from build123d import *

# Parameters (mm, degrees)
BOSS_EXTRUDE1_DEPTH      = 15
BOSS_EXTRUDE1_DEPTH_BACK = 15
SKETCH1_W                = 48
SKETCH1_H                = 65
SKETCH2_R                = 1.25
CUT_EXTRUDE1_DEPTH       = 10
SKETCH4_R                = 9.5
SKETCH4_R_2              = 8
SKETCH4_R_3              = 3
BOSS_EXTRUDE3_DEPTH      = 1.5
CHAMFER2_SIZE            = 1.5
SKETCH5_R                = 3
BOSS_EXTRUDE4_DEPTH      = 6
CHAMFER2_OF_MIRROR1_SIZE = 1.5
SKETCH6_R                = 1.25
SKETCH6_R_2              = 1.249999994
CUT_EXTRUDE2_DEPTH       = 10
FILLET1_R                = 2.5


with BuildPart() as part:
    # Sketch1 → Boss-Extrude1 (new, two sides: drawn at the far end of the back side and taken through both)
    with BuildSketch(Plane.XY.offset(-BOSS_EXTRUDE1_DEPTH_BACK)):
        Rectangle(SKETCH1_W, SKETCH1_H)
    extrude(amount=BOSS_EXTRUDE1_DEPTH + BOSS_EXTRUDE1_DEPTH_BACK)

    # Sketch2 → Cut-Extrude1 (cut)
    with BuildSketch(Plane.ZY.offset(24)):
        with Locations(Location((-12, 29.5, 0), (0, 0, 270))):
            Circle(SKETCH2_R)
        with Locations(Location((12, 29.5, 0), (0, 0, 270))):
            Circle(SKETCH2_R)
        with Locations(Location((12, 5.5, 0), (0, 0, 270))):
            Circle(SKETCH2_R)
        with Locations(Location((-12, 5.5, 0), (0, 0, 270))):
            Circle(SKETCH2_R)
        with Locations(Location((-12, -29.5, 0), (0, 0, 270))):
            Circle(SKETCH2_R)
        with Locations(Location((12, -29.5, 0), (0, 0, 270))):
            Circle(SKETCH2_R)
    extrude(amount=-CUT_EXTRUDE1_DEPTH, mode=Mode.SUBTRACT)

    # Sketch4 → Boss-Extrude3 (add)
    # profile 1 of 3: a face of its own
    with BuildSketch(Plane.ZY.offset(24)):
        with Locations(Location((0, 20.5, 0), (0, 0, 270))):
            Circle(SKETCH4_R)
        with Locations((0, 20.5)):
            Circle(SKETCH4_R_2, mode=Mode.SUBTRACT)
    # profile 2 of 3: a face of its own
    with BuildSketch(Plane.ZY.offset(24)):
        with Locations((0, 20.5)):
            Circle(SKETCH4_R_2)
        with Locations((0, 20.5)):
            Circle(SKETCH4_R_3, mode=Mode.SUBTRACT)
    # profile 3 of 3: a face of its own
    with BuildSketch(Plane.ZY.offset(24)):
        with Locations((0, 20.5)):
            Circle(SKETCH4_R_3)
    boss_extrude3 = extrude(amount=BOSS_EXTRUDE3_DEPTH)

    # Chamfer2
    chamfer2_edges = [part.edges().sort_by_distance(p)[0] for p in [
        (-25.5, 30, 0),
    ]]
    chamfer(chamfer2_edges, length=CHAMFER2_SIZE - 0.0001)  # a hair under: the kernel refuses the full size

    # Sketch5 → Boss-Extrude4 (add)
    with BuildSketch(Plane.ZY.offset(25.5)):
        with Locations(Location((0, 20.5, 0), (0, 0, 270))):
            Circle(SKETCH5_R)
    boss_extrude4 = extrude(amount=BOSS_EXTRUDE4_DEPTH)

    # Mirror1: Boss-Extrude3, Boss-Extrude4 across plane
    add(boss_extrude3.mirror(Plane(origin=(0, 0, 0), x_dir=(0, 0, 1), z_dir=(1, 0, 0))))
    add(boss_extrude4.mirror(Plane(origin=(0, 0, 0), x_dir=(0, 0, 1), z_dir=(1, 0, 0))))

    # Chamfer2 of Mirror1
    chamfer2_of_mirror1_edges = [part.edges().sort_by_distance(p)[0] for p in [
        (25.5, 30, 0),
    ]]
    chamfer(chamfer2_of_mirror1_edges, length=CHAMFER2_OF_MIRROR1_SIZE - 0.0001)  # a hair under: the kernel refuses the full size

    # Sketch6 → Cut-Extrude2 (cut)
    with BuildSketch(Plane(origin=(24, 0, 0), x_dir=(0, 0, -1), z_dir=(1, 0, 0))):
        with Locations(Location((11.99999998, -5, 0), (0, 0, 90))):
            Circle(SKETCH6_R)
        with Locations(Location((12.00000002, -17.5, 0), (0, 0, 90))):
            Circle(SKETCH6_R)
        with Locations(Location((0, -29.5, 0), (0, 0, 90))):
            Circle(SKETCH6_R_2)
        with Locations(Location((-12.00000002, -17.5, 0), (0, 0, 90))):
            Circle(SKETCH6_R)
        with Locations(Location((-12.00000002, 9.5, 0), (0, 0, 90))):
            Circle(SKETCH6_R)
    extrude(amount=-CUT_EXTRUDE2_DEPTH, mode=Mode.SUBTRACT)

    # Fillet1
    fillet1_edges = [part.edges().sort_by_distance(p)[0] for p in [
        (0, -32.5, 15),
        (0, 32.5, 15),
        (0, 32.5, -15),
        (0, -32.5, -15),
    ]]
    fillet(fillet1_edges, radius=FILLET1_R)


solid = part.part
Verification items for the finished model (mm, model axes). A direction names the side the tool comes from. Give positions to 0.01 mm unless a question says otherwise; leave off trailing zeros. Write each loop counter-clockwise with the first axis right and the second up, starting at its lowest first coordinate (ties: lowest second). Pieces come first, ordered by that corner, then holes. Notation, with made-up numbers: M -13.75,40.25 L 20.25,40.25 A34 ccw 20.25,70.25 Z; hole C 11,44.25 d3. An arc over 180 degrees is marked long. Write item = value, one per line.
(1) Material ranges on line 1 (Z direction, x = 21, y = -17.5); line 2 (X direction, y = 4, z = -6.25); line 3 (X direction, y = 23, z = 3), recorded low to high.
Found:
line_1 = -15 to -13.25, -10.75 to 10.75, 13.25 to 15
line_2 = -24 to 24
line_3 = -25.5 to 25.5
(2) Sectioned sample at A-A (y = -5). Record the cut outline in (x, z), then the cut area to 4 significant figures.
Found:
outline = M -24,-15 L 24,-15 L 24,-13.25 L 14,-13.25 L 14,-10.75 L 24,-10.75 L 24,15 L -24,15 Z
area = 1,415 mm2
(3) Sectioned sample at B-B (x = -18). Record the cut outline in (y, z).
Found:
outline = M -32.5,-12.5 A2.5 ccw -30,-15 L 30,-15 A2.5 ccw 32.5,-12.5 L 32.5,12.5 A2.5 ccw 30,15 L -30,15 A2.5 ccw -32.5,12.5 Z; hole C -29.5,-12 d2.5; hole C -29.5,12 d2.5; hole C 5.5,-12 d2.5; hole C 5.5,12 d2.5; hole C 29.5,-12 d2.5; hole C 29.5,12 d2.5
(4) Go/stop test with flat-tipped pins: pin 1 Ø3 at (y, z) = (-29.5, 0) entering from +X; pin 2 Ø0.8 at (y, z) = (5.5, 12) entering from -X; pin 3 Ø1.5 at (y, z) = (-17.5, -12) entering from -X. Record where each tip stops, or that it passes through.
Found:
pin_1 = 24
pin_2 = -14
pin_3 = -24
(5) Access from +Z, -Z, +X, -X, +Y, -Y to the whole of each face (thin tool, end or side, straight path). Record for faces 1 (the face through (14, -18, 12)), 2 (the face through (-19.07, 5.66, -10.76)), 3 (the face through (0, 0, -15)).
Found:
face_1 = +X
face_2 = -X
face_3 = -Z, +X, -X, +Y, -Y
(6) Sectioned sample at C-C (y = -17.5). Record the cut outline in (x, z), then the cut area to 3 significant figures.
Found:
outline = M -24,-15 L 24,-15 L 24,-13.25 L 14,-13.25 L 14,-10.75 L 24,-10.75 L 24,10.75 L 14,10.75 L 14,13.25 L 24,13.25 L 24,15 L -24,15 Z
area = 1,390 mm2
(7) Draft check along Z on faces 4 (the face through (14, -5, -12)), 5 (the face through (25.5, 20.6, -3.4)), 6 (the face through (25, 29, 0)), 7 (the face through (19.07, -16.345, 11.521)). Enter one of: released by +Z, released by -Z, zero draft, split by the parting line, or undercut.
Found:
face_4 = undercut
face_5 = zero draft
face_6 = split by the parting line
face_7 = undercut
